Design review of the part built by this model. Coordinates are the model's own, in mm. Face numbers are marked on the shaded views. Coordinates: 2 decimals unless noted, no trailing zeros. Loops run counter-clockwise (first coordinate to the right, second up) from the corner with the lowest first, then second, coordinate; pieces in that order, holes last. Notation, with made-up numbers: (76.5, 83.25) - (129.5, 83.25) arc R21 cw to (129.5, 94.25) - close; hole circle Ø4 at (71.25, -9.5). An arc over 180 degrees is marked (long way). One line per question, with ' | ' between items.
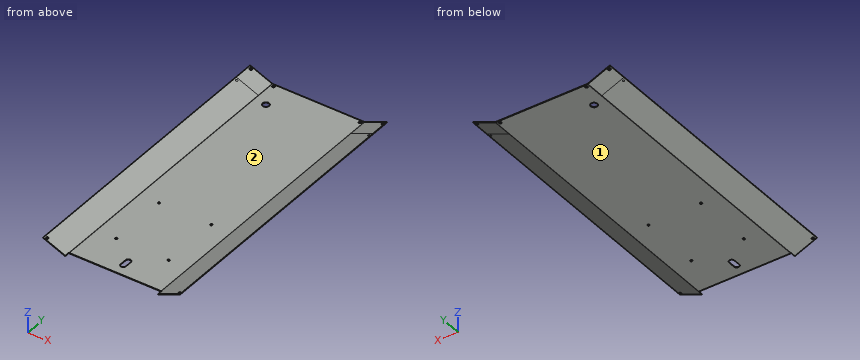
Autodesk Inventor part; units mm, degrees
ref_plane "YZ Plane" through (0, 0, 0) normal (1, 0, 0) x (0, 1, 0)
ref_plane "XZ Plane" through (0, 0, 0) normal (0, 1, 0) x (-1, 0, 0)
ref_plane "XY Plane" through (0, 0, 0) normal (0, 0, 1) x (1, 0, 0)
sketch "Sketch1" plane through (0, 0, 0) normal (0, 0, 1) x (1, 0, 0)
  line L0 (0, 0) -> (113.5, 0)
  line L1 (113.5, 0) -> (113.5, 338.525)
  line L2 (113.5, 338.525) -> (0, 338.525)
  line L3 (0, 338.525) -> (0, 0)
  dimension "d0" = 113.5
  dimension "d1" = 338.525
extrude "Plate1" add sketch "Sketch1" along normal blind 0.5
sketch "Sketch2" plane through (114.0764, 338.525, 0.6152) normal (0.3842953, 0, -0.9232102) x (0, 1, 0)
  line L0 (-338.525, 0) -> (0, 0)
  line L1 (0, 0) -> (0, 29.6214)
  line L2 (0, 29.6214) -> (-338.525, 29.6214)
  line L3 (-338.525, 29.6214) -> (-338.525, 0)
edge flange "Flange1" height 30.021 angle 22.6 thickness 0.5 bend radius 1.5 thickness toward (0.3842953, 0, -0.9232102) relief tear relief width 0.5 relief depth 0.25 edges at (113.5, 169.2625, 0.5) wall of the first edge with corners at (114.0764, 0, 0.6152) (114.0764, 338.525, 0.6152) (141.4232, 338.525, 11.9985) (141.4232, 0, 11.9985)
bend "Bend1"
corner "Corner1"
sketch "Sketch3" plane through (-0.5764, 0, 0.6152) normal (-0.3842953, 0, -0.9232102) x (0, -1, 0)
  line L0 (-338.525, 0) -> (0, 0)
  line L1 (0, 0) -> (0, 29.6214)
  line L2 (0, 29.6214) -> (-338.525, 29.6214)
  line L3 (-338.525, 29.6214) -> (-338.525, 0)
edge flange "Flange2" height 30.021 angle 22.6 thickness 0.5 bend radius 1.5 thickness toward (-0.3842953, 0, -0.9232102) relief tear relief width 0.5 relief depth 0.25 edges at (0, 169.2625, 0.5) wall of the first edge with corners at (-0.5764, 338.525, 0.6152) (-0.5764, 0, 0.6152) (-27.9232, 0, 11.9985) (-27.9232, 338.525, 11.9985)
bend "Bend2"
corner "Corner2"
sketch "Sketch4" plane through (-27.9232, 0, 11.9985) normal (0.3842953, 0, 0.9232102) x (0.9232102, 0, -0.3842953)
  line L0 (0, 338.525) -> (0, 0)
  line L1 (0, 338.525) -> (0, 335.35) construction
  line L2 (0, 335.35) -> (3.175, 335.35) construction
  circle A0 centre (3.175, 335.35) radius 1.25
  line L3 (0, 0) -> (0, 3.175) construction
  line L4 (0, 3.175) -> (3.175, 3.175) construction
  line L5 (3.175, 3.175) -> (3.175, 3.35) construction
  circle A1 centre (3.175, 3.35) radius 1.25
  point P0 (30.39, 0)
  dimension "d23" = 3.175
  dimension "d24" = 3.175
  dimension "d25" = 2.5
  dimension "d26" = 3.175
  dimension "d27" = 3.175
  dimension "d62" = 0.175
  dimension "d63" = 2.5
extrude "Extrusion1" cut sketch "Sketch4" against normal blind 10
sketch "Sketch5" plane through (0, 0, 0.5) normal (0, 0, 1) x (1, 0, 0)
  line L0 (0, 0) -> (0, 338.525)
  line L1 (113.5, 0) -> (0, 0)
  line L2 (113.5, 338.525) -> (113.5, 0)
  line L3 (0, 338.525) -> (0, 335.35) construction
  line L4 (0, 335.35) -> (3.175, 335.35) construction
  line L5 (113.5, 338.525) -> (113.5, 335.35) construction
  line L6 (113.5, 335.35) -> (110.325, 335.35) construction
  line L7 (0, 0) -> (3.175, 0) construction
  line L8 (0, 0) -> (113.5, 0) construction
  line L9 (3.175, 0) -> (3.175, 3.175) construction
  line L10 (113.5, 0) -> (113.5, 3.175) construction
  line L11 (113.5, 3.175) -> (110.325, 3.175) construction
  circle A0 centre (3.175, 335.35) radius 1.25
  circle A1 centre (110.325, 335.35) radius 1.25
  line L12 (3.175, 3.175) -> (3.175, 3.35) construction
  line L13 (110.325, 3.175) -> (110.325, 3.35) construction
  circle A2 centre (110.325, 3.35) radius 1.25
  circle A3 centre (3.175, 3.35) radius 1.25
  dimension "d31" = 3.175
  dimension "d32" = 3.175
  dimension "d33" = 3.175
  dimension "d34" = 3.175
  dimension "d35" = 3.175
  dimension "d36" = 3.175
  dimension "d37" = 3.175
  dimension "d38" = 3.175
  dimension "d41" = 2.5
  dimension "d42" = 2.5
  dimension "d58" = 0.175
  dimension "d59" = 0.175
  dimension "d60" = 2.5
  dimension "d61" = 2.5
extrude "Extrusion2" cut sketch "Sketch5" against normal blind 10
sketch "Sketch6" plane through (141.4232, 0, 11.9985) normal (-0.3842953, 0, 0.9232102) x (0.9232102, 0, 0.3842953)
  line L0 (0, 338.525) -> (0, 335.35) construction
  line L1 (0, 0) -> (0, 338.525) construction
  line L2 (0, 335.35) -> (-3.175, 335.35) construction
  line L3 (0, 0) -> (0, 3.175) construction
  line L4 (0, 3.175) -> (-3.175, 3.175) construction
  circle A0 centre (-3.175, 335.35) radius 1.25
  line L5 (-3.175, 3.175) -> (-3.175, 3.35) construction
  circle A1 centre (-3.175, 3.35) radius 1.25
  point P0 (-135.1743, 0)
  dimension "d45" = 3.175
  dimension "d46" = 3.175
  dimension "d47" = 3.175
  dimension "d48" = 3.175
  dimension "d50" = 2.5
  dimension "d64" = 0.175
  dimension "d65" = 2.5
extrude "Extrusion3" cut sketch "Sketch6" against normal blind 10
sketch "Sketch7" plane through (0, 0, 0.5) normal (0, 0, 1) x (1, 0, 0)
  line L0 (-71.3896, 0) -> (266.456, 0)
  line L1 (266.456, 0) -> (266.456, 0.175)
  line L2 (266.456, 0.175) -> (-71.3896, 0.175)
  line L3 (-71.3896, 0.175) -> (-71.3896, 0)
  dimension "d53" = 0.175
extrude "Extrusion4" cut sketch "Sketch7" against normal blind 100 and the other way blind 100
sketch "Sketch9" plane through (0, 0, 0.5) normal (0, 0, 1) x (1, 0, 0)
  circle A0 centre (3.175, 3.35) radius 1.25
  circle A1 centre (110.325, 3.35) radius 1.25
  line L0 (-0.5764, 0.175) -> (-0.5764, 338.525)
  line L1 (114.0764, 338.525) -> (114.0764, 0.175)
  line L2 (-0.5764, 0.175) -> (114.0764, 0.175)
  line L3 (114.0764, 0.175) -> (114.0764, 6.525)
  line L4 (114.0764, 6.525) -> (-0.5764, 6.525)
  line L5 (-0.5764, 6.525) -> (-0.5764, 0.175)
  point P0 (0, 0)
  dimension "d66" = 6.35
extrude "Extrusion5" cut sketch "Sketch9" against normal blind 10 and the other way blind 5
sketch "Sketch10" plane through (0, 0, 0.5) normal (0, 0, 1) x (1, 0, 0)
  line L0 (0, 6.525) -> (0, 338.525)
  line L1 (0, 6.525) -> (0, 54.375) construction
  line L2 (0, 54.375) -> (24.25, 54.375) construction
  circle A0 centre (24.25, 54.375) radius 1.25
  line L3 (24.25, 54.375) -> (89.25, 54.375) construction
  circle A1 centre (89.25, 54.375) radius 1.25
  line L4 (24.25, 54.375) -> (24.25, 129.375) construction
  circle A2 centre (24.25, 129.375) radius 1.25
  line L5 (24.25, 129.375) -> (89.25, 129.375) construction
  circle A3 centre (89.25, 129.375) radius 1.25
  point P0 (0, 0)
  dimension "d71" = 47.85
  dimension "d72" = 24.25
  dimension "d73" = 2.5
  dimension "d74" = 65
  dimension "d75" = 2.5
  dimension "d76" = 75
  dimension "d77" = 2.5
  dimension "d78" = 65
  dimension "d79" = 2.5
extrude "Extrusion6" cut sketch "Sketch10" against normal blind 10
sketch "Sketch11" plane through (0, 0, 0.5) normal (0, 0, 1) x (1, 0, 0)
  circle A0 centre (24.25, 54.375) radius 1.25
  line L0 (24.25, 54.375) -> (24.25, 29.425) construction
  line L1 (24.25, 29.425) -> (56.75, 29.425) construction
  line L2 (56.75, 29.425) -> (60, 29.425) construction
  line L3 (60, 29.425) -> (53.5, 29.425)
  line L4 (53.5, 29.425) -> (53.5, 20.925)
  line L5 (53.5, 20.925) -> (60, 20.925)
  line L6 (60, 20.925) -> (60, 29.425)
  circle A1 centre (56.75, 29.425) radius 3.25
  circle A2 centre (56.75, 20.925) radius 3.25
  point P0 (0, 0)
  dimension "d82" = 24.95
  dimension "d83" = 32.5
  dimension "d84" = 3.25
  dimension "d85" = 6.5
  dimension "d86" = 8.5
extrude "Extrusion7" cut sketch "Sketch11" against normal blind 10 contours A1 L3 | L3 A1 | L6 A2 L4 A1 | A2 L5 | L5 A2
sketch "Sketch13" plane through (0, 338.525, 0) normal (0, 1, 0) x (1, 0, 0)
  line L0 (0, -0.5) -> (113.5, -0.5)
  line L1 (113.5, 0) -> (113.5, -0.5)
  line L2 (113.5, 0) -> (0, 0)
  line L3 (0, 0) -> (0, -0.5)
extrude "Extrusion8" add sketch "Sketch13" along normal blind 30.87
sketch "Sketch14" plane through (-28.1153, 338.525, 11.5369) normal (0, 1, 0) x (0.9232102, 0, -0.3842953)
  line L0 (29.6214, -0.5) -> (29.6214, 0)
  line L1 (29.6214, 0) -> (0, 0)
  line L2 (0, -0.5) -> (0, 0)
  line L3 (0, -0.5) -> (29.6214, -0.5)
  point P0 (30.39, -0.1536)
extrude "Extrusion9" add sketch "Sketch14" along normal blind 30.87
sketch "Sketch15" plane through (0, 338.525, 0.5) normal (0, 1, 0) x (1, 0, 0)
  line L0 (-0.5764, -0.1152) -> (-0.7686, 0.3464)
  arc A0 (0, 0) -> (-0.5764, -0.1152) centre (0, -1.5) ccw
  line L1 (0, 0.5) -> (0, 0)
  arc A1 (0, 0.5) -> (-0.7686, 0.3464) centre (0, -1.5) ccw
extrude "Extrusion10" add sketch "Sketch15" along normal blind 30.87
sketch "Sketch16" plane through (113.5, 338.525, 0.5) normal (0, 1, 0) x (1, 0, 0)
  line L0 (0.7686, 0.3464) -> (0.5764, -0.1152)
  arc A0 (0.7686, 0.3464) -> (0, 0.5) centre (0, -1.5) ccw
  line L1 (0, 0.5) -> (0, 0)
  arc A1 (0.5764, -0.1152) -> (0, 0) centre (0, -1.5) ccw
  point P0 (-113.5, 0.5)
extrude "Extrusion11" add sketch "Sketch16" along normal blind 30.87
sketch "Sketch17" plane through (114.0764, 338.525, 0.6152) normal (0, 1, 0) x (0.9232102, 0, 0.3842953)
  line L0 (0, 0.5) -> (0, 0)
  line L1 (29.6214, 0) -> (0, 0)
  line L2 (29.6214, 0) -> (29.6214, 0.5)
  line L3 (29.6214, 0.5) -> (0, 0.5)
  point P0 (-105.553, -43.2711)
extrude "Extrusion12" add sketch "Sketch17" along normal blind 30.87
sketch "Sketch18" plane through (-27.9232, 0.175, 11.9985) normal (0.3842953, 0, 0.9232102) x (0.9232102, 0, -0.3842953)
  circle A0 centre (3.175, 335.175) radius 1.25
  circle A1 centre (3.175, 335.175) radius 1.25
  point P0 (30.39, -0.175)
  dimension "d100" = 2.5
extrude "Extrusion13" add sketch "Sketch18" against normal up to surface (0.5 mm away)
sketch "Sketch19" plane through (0, 0, 0.5) normal (0, 0, 1) x (1, 0, 0)
  circle A0 centre (110.325, 335.35) radius 1.25
  circle A1 centre (3.175, 335.35) radius 1.25
  point P0 (0, 0)
extrude "Extrusion14" add sketch "Sketch19" against normal up to surface (0.5 mm away)
sketch "Sketch20" plane through (141.4232, 0.175, 11.9985) normal (-0.3842953, 0, 0.9232102) x (0.9232102, 0, 0.3842953)
  circle A0 centre (-3.175, 335.175) radius 1.25
  circle A1 centre (-3.175, 335.175) radius 1.25
  point P0 (-135.1743, -0.175)
extrude "Extrusion15" add sketch "Sketch20" against normal up to surface (0.5 mm away)
sketch "Sketch21" plane through (-27.9232, 0.175, 11.9985) normal (0.3842953, 0, 0.9232102) x (0.9232102, 0, -0.3842953)
  line L0 (0, 369.22) -> (0, 359.695) construction
  line L1 (0, 0) -> (0, 369.22) construction
  line L2 (0, 359.695) -> (3.175, 359.695) construction
  circle A0 centre (3.175, 359.695) radius 1.5
  point P0 (30.39, -0.175)
  dimension "d107" = 9.525
  dimension "d108" = 3.175
  dimension "d109" = 3
extrude "Extrusion16" cut sketch "Sketch21" against normal blind 30.87
sketch "Sketch22" plane through (0, 0, 0.5) normal (0, 0, 1) x (1, 0, 0)
  line L0 (113.5, 6.525) -> (113.5, 369.395)
  line L1 (0, 369.395) -> (0, 359.87) construction
  line L2 (0, 6.525) -> (0, 369.395) construction
  line L3 (0, 359.87) -> (3.175, 359.87) construction
  circle A0 centre (3.175, 359.87) radius 1.5
  line L4 (113.5, 6.525) -> (113.5, 369.395) construction
  line L5 (113.5, 369.395) -> (113.5, 359.87) construction
  line L6 (113.5, 359.87) -> (110.325, 359.87) construction
  circle A1 centre (110.325, 359.87) radius 1.5
  point P0 (0, 0)
  dimension "d112" = 9.525
  dimension "d113" = 3.175
  dimension "d114" = 3
  dimension "d115" = 9.525
  dimension "d116" = 3.175
  dimension "d117" = 3
extrude "Extrusion17" cut sketch "Sketch22" against normal blind 30.87
sketch "Sketch23" plane through (141.4232, 0.175, 11.9985) normal (-0.3842953, 0, 0.9232102) x (0.9232102, 0, 0.3842953)
  line L0 (0, 0) -> (0, 369.22)
  line L1 (0, 369.22) -> (0, 359.695) construction
  line L2 (0, 359.695) -> (-3.175, 359.695) construction
  circle A0 centre (-3.175, 359.695) radius 1.5
  point P0 (-135.1743, -0.175)
  dimension "d120" = 9.525
  dimension "d121" = 3.175
  dimension "d122" = 3
extrude "Extrusion18" cut sketch "Sketch23" against normal blind 30.87
sketch "Sketch24" plane through (0, 0, 0.5) normal (0, 0, 1) x (1, 0, 0)
  line L0 (-33.1091, 369.395) -> (215.7214, 369.395)
  line L1 (215.7214, 369.395) -> (215.7214, 363.045)
  line L2 (215.7214, 363.045) -> (-33.1091, 363.045)
  line L3 (-33.1091, 363.045) -> (-33.1091, 369.395)
  point P0 (0, 0)
  dimension "d125" = 6.35
extrude "Extrusion19" cut sketch "Sketch24" against normal blind 30.87 and the other way blind 15.435
sketch "Sketch25" plane through (0, 0, 0.5) normal (0, 0, 1) x (1, 0, 0)
  line L0 (0, 363.045) -> (0, 330.045) construction
  line L1 (0, 6.525) -> (0, 363.045) construction
  line L2 (0, 330.045) -> (15, 330.045) construction
  circle A0 centre (15, 330.045) radius 4
  point P0 (0, 0)
  dimension "d130" = 33
  dimension "d131" = 15
  dimension "d132" = 8
extrude "Extrusion20" cut sketch "Sketch25" against normal blind 10
equation "\"d2\" = Thickness"
equation "\"d3\" = BendReliefWidth"
equation "\"d4\" = BendReliefDepth"
equation "\"d5\" = MinimumRemnant"
equation "\"d6\" = TransitionRadius"
equation "\"d10\" = CornerReliefSize"
equation "\"d11\" = GapSize"
equation "\"d12\" = JacobiRadiusSize"
equation "\"d13\" = BendReliefWidth"
equation "\"d14\" = BendReliefDepth"
equation "\"d15\" = MinimumRemnant"
equation "\"d16\" = TransitionRadius"
equation "\"d20\" = CornerReliefSize"
equation "\"d21\" = GapSize"
equation "\"d22\" = JacobiRadiusSize"
equation "\"BendRadius\" = Thickness"
equation "\"BendReliefWidth\" = Thickness"
equation "\"BendReliefDepth\" = 0.5 * Thickness"
equation "\"CornerReliefSize\" = 4 * Thickness"
equation "\"MinimumRemnant\" = 2 * Thickness"
equation "\"TransitionRadius\" = BendRadius"
equation "\"JacobiRadiusSize\" = BendRadius"
equation "\"GapSize\" = Thickness"
properties part number "sideplate part 4" material "Aluminum 6061"
Q1. Take a section at D-D (x = 15). Give the boundary of the cut face in (y, z) (3 decimals), plus the area to 3 significant figures.
Returned:
outline: (6.525, 0) - (326.045, 0) - (326.045, 0.5) - (6.525, 0.5) - close; (334.045, 0) - (363.045, 0) - (363.045, 0.5) - (334.045, 0.5) - close | area: 174 mm²
Q2. Take a section at C-C (y = 61.5). Give the boundary of the cut face in (x, z).
Returned:
outline: (-28.12, 11.54) - (-0.77, 0.15) arc R2 ccw to (0, 0) - (113.5, 0) arc R2 ccw to (114.27, 0.15) - (141.62, 11.54) - (141.42, 12) - (114.08, 0.62) arc R1.5 cw to (113.5, 0.5) - (0, 0.5) arc R1.5 cw to (-0.58, 0.62) - (-27.92, 12) - close
Q3. Take a section at A-A (x = 56.75). Give the boundary of the cut face in (y, z) (3 decimals), plus the area to 3 significant figures.
Returned:
outline: (6.525, 0) - (17.675, 0) - (17.675, 0.5) - (6.525, 0.5) - close; (32.675, 0) - (363.045, 0) - (363.045, 0.5) - (32.675, 0.5) - close | area: 171 mm²
Q4. Draft analysis for pull direction X (two halves, no side actions). For the marked faces 1 and 2, state which applies: +X half, -X half, draft (parallel to the pull), parting line (faces both ways), or undercut.
Returned:
face 1: draft | face 2: undercut
Q5. To check wall thickness, follow line 1 along Y through (x, z) = (24.25, 0.3) (3 decimals); line 2 along Y through (x, z) = (15, 0.35) (3 decimals); line 3 along Z through (x, y) = (65, 247). State the ranges of each line that lie inside material, in increasing order.
Returned:
line 1: y = 6.525 to 53.125, 55.625 to 128.125, 130.625 to 363.045 | line 2: y = 6.525 to 326.045, 334.045 to 363.045 | line 3: z = 0 to 0.5
Q6. For pin 1 (10 mm diameter, centred on x = -10.5, y = 153, fed in from +Z); pin 2 (2.5 mm diameter, centred on x = 110.325, y = 359.87, fed in from -Z); pin 3 (4 mm diameter, centred on x = 89, y = 83, fed in from +Z), all flat-tipped, find the tip position at first contact; note any pin that passes through.
Returned:
pin 1: stops at z = 6.83 | pin 2: passes through | pin 3: stops at z = 0.5
Q7. Take a section at B-B (z = 2.5). Give the boundary of the cut face in (x, y) (3 decimals), plus the area to 3 significant figures.
Returned:
outline: (-6.406, 363.045) - (-6.405, 0.175) - (-5.104, 0.175) - (-5.104, 363.045) - close; (118.604, 0.175) - (119.905, 0.175) - (119.905, 363.045) - (118.604, 363.045) - close | area: 944 mm²
